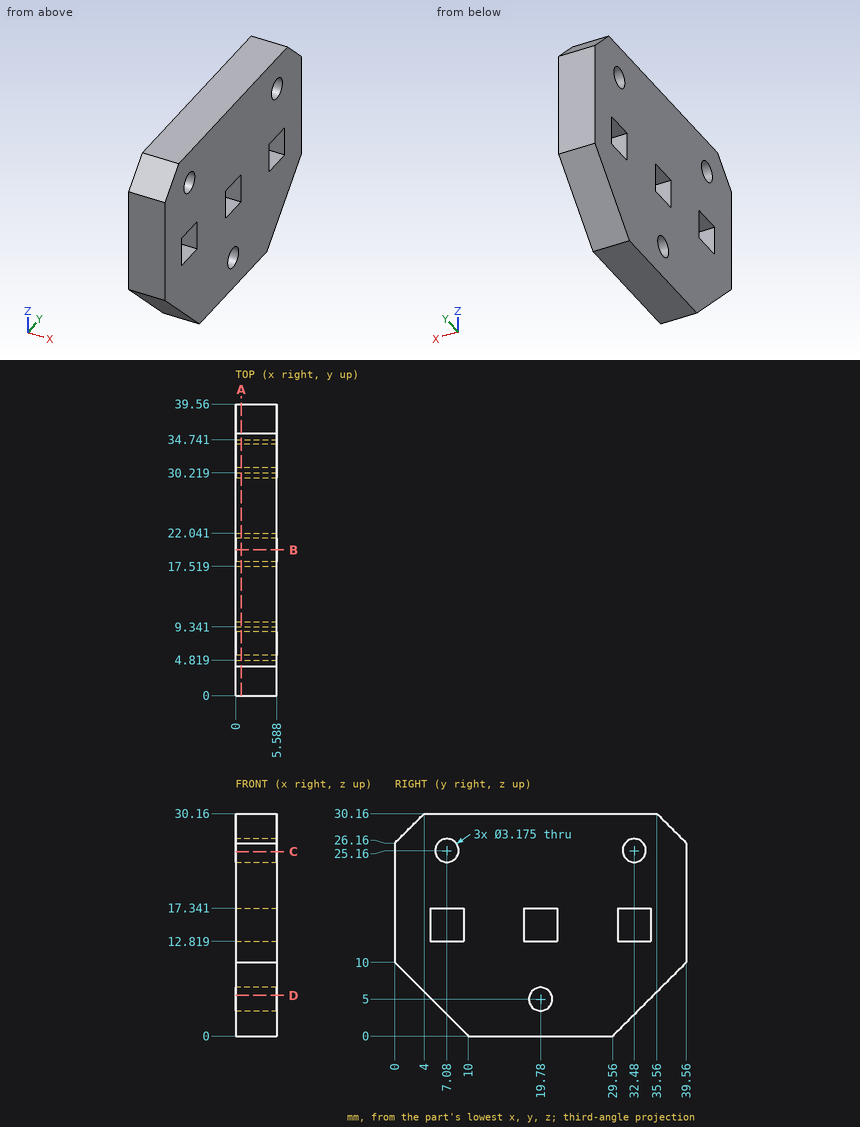
Can you work these out from the drawing? Everything is in mm from the part's minimum corner. Coordinates: 2 decimals unless noted, no trailing zeros. Order: outer loops, then holes, each group sorted by start corner. A loop starts at its lowest first (then second) coordinate and runs counter-clockwise, first axis right, second up. Notation, with made-up numbers: M 62.5,26.5 L 85.5,26.5 A24 cw 85.5,64.5 Z; hole C 15.25,57.25 d1. An arc over 180 degrees is marked long. Answer as CSV lines item,"result". Start each with the question number.
1. I need wall thicknesses on line 1 (Y direction, x = 1.4, z = 13.5); line 2 (Z direction, x = 1.8, y = 6) (1 decimal); line 3 (Z direction, x = 0.8, y = 20.5) (1 decimal). Which ranges of each line are inside material? Lowest first, please. Write a range as [from, to].
2. I want a section at C-C, the plane z = 25. Write out the boundary of the cut face in (x, y).
3. For pin 1 (4 mm diameter, centred on y = 32.48, z = 25.16, fed in from +X); pin 2 (1.4 mm diameter, centred on x = 3, y = 6.5, fed in from -Z); pin 3 (1 mm diameter, centred on x = 1.5, z = 6.5, fed in from +Y), each with a flat end and sliding along its axis, tell me the tip position at first contact or that it passes through.
4. I want a section at D-D, the plane z = 5.5. Write out the boundary of the cut face in (x, y), and give its area (3 significant figures).
5. I want a section at B-B, the plane y = 19.78. Write out the boundary of the cut face in (x, z).
6. I want a section at A-A, the plane x = 0.8. Write out the boundary of the cut face in (y, z) (1 decimal), and give its area (3 significant figures).
Recorded:
1,line 1,"y = [0, 4.82], [9.34, 17.52], [22.04, 30.22], [34.74, 39.56]"
1,line 2,"z = [4, 12.8], [17.3, 24], [26.3, 30.2]"
1,line 3,"z = [0, 3.6], [6.4, 12.8], [17.3, 30.2]"
2,outline,"M 0,0 L 5.59,0 L 5.59,5.5 L 0,5.5 Z; M 0,8.66 L 5.59,8.66 L 5.59,30.9 L 0,30.9 Z; M 0,34.06 L 5.59,34.06 L 5.59,39.56 L 0,39.56 Z"
3,pin 1,"stops at x = 5.59"
3,pin 2,"stops at z = 2.8"
3,pin 3,"stops at y = 36.56"
4,outline,"M 0,4.5 L 5.59,4.5 L 5.59,18.27 L 0,18.27 Z; M 0,21.29 L 5.59,21.29 L 5.59,35.06 L 0,35.06 Z"
4,area,"154 mm2"
5,outline,"M 0,0 L 5.59,0 L 5.59,3.41 L 0,3.41 Z; M 0,6.59 L 5.59,6.59 L 5.59,12.82 L 0,12.82 Z; M 0,17.34 L 5.59,17.34 L 5.59,30.16 L 0,30.16 Z"
6,outline,"M 0,10 L 10,0 L 29.6,0 L 39.6,10 L 39.6,26.2 L 35.6,30.2 L 4,30.2 L 0,26.2 Z; hole M 4.8,12.8 L 9.3,12.8 L 9.3,17.3 L 4.8,17.3 Z; hole C 7.1,25.2 d3.2; hole M 17.5,12.8 L 22,12.8 L 22,17.3 L 17.5,17.3 Z; hole C 19.8,5 d3.2; hole M 30.2,12.8 L 34.7,12.8 L 34.7,17.3 L 30.2,17.3 Z; hole C 32.5,25.2 d3.2"
6,area,"992 mm2"
